from build123d import *

# Parameters (mm, degrees)
BOSS_EXTRUDE1_DEPTH = 38.1
SKETCH7_W           = 6.35
SKETCH7_H           = 101.6
SKETCH7_H_2         = 100.875432805
CUT_EXTRUDE1_DEPTH  = 140.9883388
CIRPATTERN1_COUNT   = 4


with BuildPart() as part:
    # Sketch1 → Boss-Extrude1 (new body)
    with BuildSketch(Plane(origin=(0, 0, 0), x_dir=(1, 0, 0), z_dir=(0, 1, 0))):
        with BuildLine():
            Line((-33.444507811, 89.185354163), (-33.444507811, 33.696150168))
            Line((-33.444507811, 33.696150168), (-89.090582913, 33.696150168))
            ThreePointArc((-89.090582913, 33.696150168), (-95.25, 0), (-89.090582913, -33.696150168))
            Line((-89.090582913, -33.696150168), (-33.444507811, -33.696150168))
            Line((-33.444507811, -33.696150168), (-33.444507811, -89.185354163))
            ThreePointArc((-33.444507811, -89.185354163), (0, -95.25), (33.444507811, -89.185354163))
            Line((33.444507811, -89.185354163), (33.444507811, -33.696150168))
            Line((33.444507811, -33.696150168), (89.090582913, -33.696150168))
            ThreePointArc((89.090582913, -33.696150168), (95.25, 0), (89.090582913, 33.696150168))
            Line((89.090582913, 33.696150168), (33.444507811, 33.696150168))
            Line((33.444507811, 33.696150168), (33.444507811, 89.185354163))
            ThreePointArc((33.444507811, 89.185354163), (0, 95.25), (-33.444507811, 89.185354163))
        make_face()
    extrude(amount=-BOSS_EXTRUDE1_DEPTH)

    # Sketch3 → Cut-Revolve3 (revolve, cut)
    with BuildSketch(Plane.XY.offset(59.69)):
        with BuildLine():
            Line((0, 0), (0, -31.75))
            ThreePointArc((0, -31.75), (22.450640303, -22.450640303), (31.75, 0))
            Line((31.75, 0), (0, 0))
        make_face()
    cut_revolve3 = revolve(axis=Axis((0, 0, 59.69), (0, -1, 0)), mode=Mode.SUBTRACT)

    # Sketch7 → Cut-Extrude1 (cut, through all)
    with BuildSketch(Plane(origin=(0, 0, 0), x_dir=(1, 0, 0), z_dir=(0, 1, 0))):
        with Locations((-16.256, -76.2)):
            Rectangle(SKETCH7_W, SKETCH7_H)
        with Locations((0, -76.2)):
            Rectangle(SKETCH7_W, SKETCH7_H)
        with Locations((16.256, -75.837716403)):
            Rectangle(SKETCH7_W, SKETCH7_H_2)
        with Locations((36.576, -76.171178844)):
            Rectangle(SKETCH7_W, SKETCH7_H)
        with Locations((-36.576, -76.2)):
            Rectangle(SKETCH7_W, SKETCH7_H)
    cut_extrude1 = extrude(amount=-CUT_EXTRUDE1_DEPTH, mode=Mode.SUBTRACT)

    # CirPattern1: Cut-Revolve3, Cut-Extrude1 ×4 about axis
    cirpattern1_axis = Axis((0, 0, 0), (0, 1, 0))
    add([cut_revolve3.rotate(cirpattern1_axis, i * 360 / CIRPATTERN1_COUNT) for i in range(1, CIRPATTERN1_COUNT)], mode=Mode.SUBTRACT)
    add([cut_extrude1.rotate(cirpattern1_axis, i * 360 / CIRPATTERN1_COUNT) for i in range(1, CIRPATTERN1_COUNT)], mode=Mode.SUBTRACT)


solid = part.part
Model file for the job. Use its own axes, mm. A direction names the side the tool comes from. Give positions to 0.01 mm unless a question says otherwise; leave off trailing zeros. Order: outer loops, then holes, each group sorted by start corner. A loop starts at its lowest first (then second) coordinate and runs counter-clockwise, first axis right, second up. Notation, with made-up numbers: (33.5, 73.5) - (60.5, 73.5) arc R8 ccw to (60.5, 87.5) - close; hole circle Ø6 at (44.25, 72.25). An arc over 180 degrees is marked (long way). Return JSON: item names as keys, results as strings.
1) Cut at B-B, the plane z = -80.5. Give the cut face in (x, y) (3 decimals).
Geometry says:
{"outline": "(-33.401, -38.1) - (-19.431, -38.1) - (-19.431, -14.051) arc R23.979 cw to (-23.979, 0) - (-33.401, 0) - close; (-13.081, -38.1) - (-3.175, -38.1) - (-3.175, -23.768) arc R23.979 cw to (-13.081, -20.097) - close; (3.175, -38.1) - (13.081, -38.1) - (13.081, -20.097) arc R23.979 cw to (3.175, -23.768) - close; (19.431, -38.1) - (33.401, -38.1) - (33.401, 0) - (23.979, 0) arc R23.979 cw to (19.431, -14.051) - close"}
2) Cut at D-D, the plane z = -10. Give the cut face in (x, y), plus the area to 3 significant figures.
Geometry says:
{"outline": "(-94.72, -38.1) - (94.72, -38.1) - (94.72, 0) - (89.82, 0) arc R30.13 cw to (29.56, 0) - (-29.56, 0) arc R30.13 cw to (-89.82, 0) - (-94.72, 0) - close", "area": "4,370 mm²"}
3) Cut at A-A, the plane x = -63.5. Give the cut face in (y, z) (3 decimals), plus the area to 3 significant figures.
Geometry says:
{"outline": "(-38.1, -33.401) - (0, -33.401) - (0, -31.521) arc R31.521 cw to (-24.819, -19.431) - (-38.1, -19.431) - close; (-38.1, -13.081) - (-28.678, -13.081) arc R31.521 cw to (-31.36, -3.175) - (-38.1, -3.175) - close; (-38.1, 3.175) - (-31.36, 3.175) arc R31.521 cw to (-28.678, 13.081) - (-38.1, 13.081) - close; (-38.1, 19.431) - (-24.819, 19.431) arc R31.521 cw to (0, 31.521) - (0, 33.401) - (-38.1, 33.401) - close", "area": "800 mm²"}
4) Probe line 1 (X direction, y = -28, z = 83.5) (3 decimals); line 2 (Z direction, x = 44, y = -21.5). List the from-to ranges inside material, lowest first. Write a range as from..to.
Geometry says:
{"line 1": "-33.401..-19.431, -13.081..-3.175, 3.175..13.081, 19.431..33.401", "line 2": "-33.4..-19.43, 19.43..33.4"}
5) Pull direction Z, two halves, no side cores. Call faces 1 (the flat face through (-13.081, -31, -60)), 2 (the flat face through (-37, -19, 25.4)), 3 (the flat face through (25.4, -19, -16)), 4 (the flat face through (25.4, -19, 16)): pulls with the +Z half, pulls with the -Z half, needs draft (parallel to the pull), parting line crosses it, or undercut.
Geometry says:
{"face 1": "needs draft", "face 2": "pulls with the +Z half", "face 3": "undercut", "face 4": "undercut"}
6) Flat gauge pins, fed straight in: P1, Ø19, axis at x = -60, y = -17.5, coming from the -Z side; P2, Ø9, axis at y = -17, z = 29, coming from the +X side; P3, Ø3, axis at x = -17.5, y = -23.5, coming from the +Z side. Where does each tip first touch, or does it go through?
Geometry says:
{"P1": "z = -33.4", "P2": "x = 92.05", "P3": "z = 25.4"}
7) 3-axis set-ups, long thin cutter, end or side, ignore diameter. For faces 5 (the flat face through (13.081, -31, -60)), 6 (the flat face through (65, -19, 33.401)), 7 (the flat face through (60, -27, 19.431)), 8 (the flat face through (37, -19, 25.371)), 9 (the flat face through (-25.371, -19, 37)): which of +Z, -Z, +X, -X, +Y, -Y reach the whole face in a straight line?
Geometry says:
{"face 5": "-Z, +Y, -Y", "face 6": "+Z, +X, +Y, -Y", "face 7": "+X, +Y, -Y", "face 8": "+Z, +Y, -Y", "face 9": "-X, +Y, -Y"}
8) Cut at C-C, the plane y = -12. Count the separate pieces of the cut face and the enclosed holes in it, plus the area to 3 significant figures.
Geometry says:
{"separate pieces": "9", "enclosed holes": "0", "area": "7,910 mm²"}
